from build123d import *

# Parameters (mm, degrees)
SKETCH1_R           = 12.7
SKETCH1_R_2         = 11.049
BOSS_EXTRUDE1_DEPTH = 242
SKETCH2_R           = 1.6
CUT_EXTRUDE1_DEPTH  = 13.7


with BuildPart() as part:
    # Sketch1 → Boss-Extrude1 (new body, symmetric)
    with BuildSketch(Plane.XY):
        Circle(SKETCH1_R)
        Circle(SKETCH1_R_2, mode=Mode.SUBTRACT)
    extrude(amount=BOSS_EXTRUDE1_DEPTH, both=True)

    # Sketch2 → Cut-Extrude1 (cut, symmetric)
    with BuildSketch(Plane(origin=(0, 0, 0), x_dir=(1, 0, 0), z_dir=(0, 1, 0))):
        with Locations((0, -232)):
            Circle(SKETCH2_R)
    cut_extrude1 = extrude(amount=CUT_EXTRUDE1_DEPTH, both=True, mode=Mode.SUBTRACT)

    # Mirror1: Cut-Extrude1 across plane
    add(cut_extrude1.mirror(Plane.XY), mode=Mode.SUBTRACT)


solid = part.part
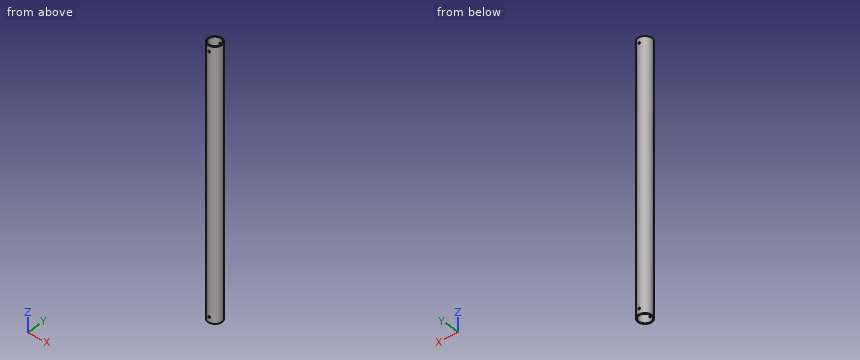
Geometry: final body of the model. Coordinates: model frame, mm. Round coordinates to 2 decimals unless told otherwise and drop trailing zeros. Loops run counter-clockwise (first coordinate to the right, second up) from the corner with the lowest first, then second, coordinate; pieces in that order, holes last. Notation, with made-up numbers: (67, -15) - (103, -15) arc R29 ccw to (103, 8) - close; hole circle Ø6 at (-6, 81). An arc over 180 degrees is marked (long way). Write each question's results on one line, items separated by ' | '. Start each with the question number.
1) Cut plane A-A on y = 0. Return loops of the section in (x, z), then the cut area to 3 significant figures.
2) Line query: probe 1 along Z at (x, y) = (0, 12.25); probe 2 along Y at (x, z) = (0, -55); probe 3 along X at (y, z) = (3.75, -214.5). Output: solid intervals per line, ascending. Write a range as [from, to].
3) Cut plane B-B on x = -6.5. Return loops of the section in (y, z), then the cut area to 3 significant figures.
4) First-contact query: P1, Ø1.9, axis at x = 0, z = 232, coming from the -Y side; P2, Ø8, axis at x = 9, z = -117, coming from the +Y side; P3, Ø3, axis at x = 0.5, z = -74.5, coming from the +Y side; P4, Ø6, axis at y = 3.5, z = 14, coming from the +X side. Flat tips, straight axial feed; report the tip coordinate or a pass-through.
5) Cut plane C-C on z = 62. Return loops of the section in (x, y), then the cut area to 3 significant figures.
Verdict:
1) outline: (-12.7, -242) - (-11.05, -242) - (-11.05, 242) - (-12.7, 242) - close; (11.05, -242) - (12.7, -242) - (12.7, 242) - (11.05, 242) - close | area: 1,600 mm2
2) probe 1: z = [-242, -233.6], [-230.4, 230.4], [233.6, 242] | probe 2: y = [-12.7, -11.05], [11.05, 12.7] | probe 3: x = [-12.13, -10.39], [10.39, 12.13]
3) outline: (-10.91, -242) - (-8.93, -242) - (-8.93, 242) - (-10.91, 242) - close; (8.93, -242) - (10.91, -242) - (10.91, 242) - (8.93, 242) - close | area: 1,910 mm2
4) P1: passes through | P2: stops at y = 11.67 | P3: stops at y = 12.7 | P4: stops at x = 12.69
5) outline: circle Ø25.4 at (0, 0); hole circle Ø22.1 at (0, 0) | area: 123 mm2
